```python
from build123d import *

# Parameters (mm, degrees)
EXTRUDE_1_DEPTH          = 660
CUT_EXTRUDE_1_DEPTH      = 661
CUT_EXTRUDE_1_DEPTH_BACK = 661
SHELL_1_T                = 10


with BuildPart() as part:
    # 草图1 → 凸台-拉伸1 (new body, symmetric)
    with BuildSketch(Plane(origin=(0, 0, 0), x_dir=(1, 0, 0), z_dir=(0, 1, 0))):
        Polygon((395, 8.660254038), (205, 337.749907476), (190, 346.410161514), (-190, 346.410161514), (-205, 337.749907476), (-395, 8.660254038), (-395, -8.660254038), (-205, -337.749907476), (-190, -346.410161514), (190, -346.410161514), (205, -337.749907476), (395, -8.660254038), align=None)
    extrude(amount=EXTRUDE_1_DEPTH, both=True)

    # 草图4 → 切除-拉伸1 (cut, two sides)
    with BuildSketch(Plane(origin=(0, 0, 0), x_dir=(1, 0, 0), z_dir=(0, 1, 0))) as cut_extrude_1_sk:
        with BuildLine():
            Line((190, 369.620348729), (190, 346.410161514))
            Line((190, 346.410161514), (11.76, 310.784114995))
            ThreePointArc((11.76, 310.784114995), (0, 309.620348729), (-11.76, 310.784114995))
            Line((-11.76, 310.784114995), (-190, 346.410161514))
            Line((-190, 346.410161514), (-190, 369.620348729))
            Line((-190, 369.620348729), (-190, 392.830535944))
            Line((-190, 392.830535944), (-11.76, 428.456582463))
            ThreePointArc((-11.76, 428.456582463), (0, 429.620348729), (11.76, 428.456582463))
            Line((11.76, 428.456582463), (190, 392.830535944))
            Line((190, 392.830535944), (190, 369.620348729))
        make_face()
        with BuildLine():
            Line((415.100611755, 20.265347645), (395, 8.660254038))
            Line((395, 8.660254038), (275.026938678, 145.207598749))
            ThreePointArc((275.026938678, 145.207598749), (268.139087528, 154.810174364), (263.266938678, 165.576516246))
            Line((263.266938678, 165.576516246), (205, 337.749907476))
            Line((205, 337.749907476), (225.100611755, 349.355001084))
            Line((225.100611755, 349.355001084), (245.20122351, 360.960094691))
            Line((245.20122351, 360.960094691), (365.174284832, 224.41274998))
            ThreePointArc((365.174284832, 224.41274998), (372.062135982, 214.810174364), (376.934284832, 204.043832483))
            Line((376.934284832, 204.043832483), (435.20122351, 31.870441253))
            Line((435.20122351, 31.870441253), (415.100611755, 20.265347645))
        make_face()
        with BuildLine():
            Line((225.100611755, -349.355001084), (205, -337.749907476))
            Line((205, -337.749907476), (263.266938678, -165.576516246))
            ThreePointArc((263.266938678, -165.576516246), (268.139087528, -154.810174364), (275.026938678, -145.207598749))
            Line((275.026938678, -145.207598749), (395, -8.660254038))
            Line((395, -8.660254038), (415.100611755, -20.265347645))
            Line((415.100611755, -20.265347645), (435.20122351, -31.870441253))
            Line((435.20122351, -31.870441253), (376.934284832, -204.043832483))
            ThreePointArc((376.934284832, -204.043832483), (372.062135982, -214.810174364), (365.174284832, -224.41274998))
            Line((365.174284832, -224.41274998), (245.20122351, -360.960094691))
            Line((245.20122351, -360.960094691), (225.100611755, -349.355001084))
        make_face()
        with BuildLine():
            Line((-190, -369.620348729), (-190, -346.410161514))
            Line((-190, -346.410161514), (-11.76, -310.784114995))
            ThreePointArc((-11.76, -310.784114995), (0, -309.620348729), (11.76, -310.784114995))
            Line((11.76, -310.784114995), (190, -346.410161514))
            Line((190, -346.410161514), (190, -369.620348729))
            Line((190, -369.620348729), (190, -392.830535944))
            Line((190, -392.830535944), (11.76, -428.456582463))
            ThreePointArc((11.76, -428.456582463), (0, -429.620348729), (-11.76, -428.456582463))
            Line((-11.76, -428.456582463), (-190, -392.830535944))
            Line((-190, -392.830535944), (-190, -369.620348729))
        make_face()
        with BuildLine():
            Line((-415.100611755, -20.265347645), (-395, -8.660254038))
            Line((-395, -8.660254038), (-275.026938678, -145.207598749))
            ThreePointArc((-275.026938678, -145.207598749), (-268.139087528, -154.810174364), (-263.266938678, -165.576516246))
            Line((-263.266938678, -165.576516246), (-205, -337.749907476))
            Line((-205, -337.749907476), (-225.100611755, -349.355001084))
            Line((-225.100611755, -349.355001084), (-245.20122351, -360.960094691))
            Line((-245.20122351, -360.960094691), (-365.174284832, -224.41274998))
            ThreePointArc((-365.174284832, -224.41274998), (-372.062135982, -214.810174364), (-376.934284832, -204.043832483))
            Line((-376.934284832, -204.043832483), (-435.20122351, -31.870441253))
            Line((-435.20122351, -31.870441253), (-415.100611755, -20.265347645))
        make_face()
        with BuildLine():
            Line((-225.100611755, 349.355001084), (-205, 337.749907476))
            Line((-205, 337.749907476), (-263.266938678, 165.576516246))
            ThreePointArc((-263.266938678, 165.576516246), (-268.139087528, 154.810174364), (-275.026938678, 145.207598749))
            Line((-275.026938678, 145.207598749), (-395, 8.660254038))
            Line((-395, 8.660254038), (-415.100611755, 20.265347645))
            Line((-415.100611755, 20.265347645), (-435.20122351, 31.870441253))
            Line((-435.20122351, 31.870441253), (-376.934284832, 204.043832483))
            ThreePointArc((-376.934284832, 204.043832483), (-372.062135982, 214.810174364), (-365.174284832, 224.41274998))
            Line((-365.174284832, 224.41274998), (-245.20122351, 360.960094691))
            Line((-245.20122351, 360.960094691), (-225.100611755, 349.355001084))
        make_face()
    extrude(amount=CUT_EXTRUDE_1_DEPTH, mode=Mode.SUBTRACT)
    extrude(cut_extrude_1_sk.sketch, amount=-CUT_EXTRUDE_1_DEPTH_BACK, mode=Mode.SUBTRACT)

    # 抽壳1 (no face opened: a closed hollow body)
    add(offset(amount=-SHELL_1_T, mode=Mode.PRIVATE), mode=Mode.SUBTRACT)


solid = part.part
```
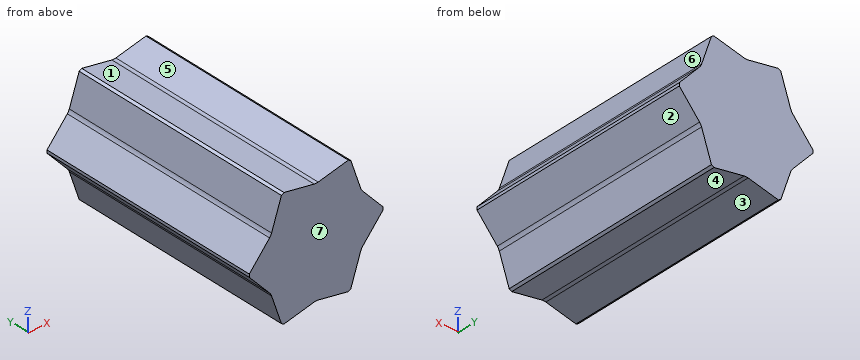
Check sheet for the modelled part. Datum: model origin and axes. Units: mm. Face numbers are marked on the shaded views. A direction names the side the tool comes from. Give positions to 0.01 mm unless a question says otherwise; leave off trailing zeros. Order: outer loops, then holes, each group sorted by start corner. A loop starts at its lowest first (then second) coordinate and runs counter-clockwise, first axis right, second up. Notation, with made-up numbers: (-22.75, -35.5) -> (-14.75, -35.5) arc R19 ccw to (-14.75, -9.5) -> close; hole circle Ø3 at (29, 0.25). An arc over 180 degrees is marked (long way). Use CSV: the item, a comma, the result in double quotes. Start each with the question number.
1) Material ranges on line 1 (Y direction, x = 195.5, z = -177.5); line 2 (X direction, y = 77, z = 289); line 3 (X direction, y = -560, z = 197), recorded low to high. Write a range as from..to.
2) Mould release check, pull along X, two halves, no side actions. Record for the marked faces 4, 5, 6 and 7: released by +X, released by -X, zero draft, split by the parting line, or undercut.
3) Set-up check for the marked faces 1, 2 and 3: record each of +Z, -Z, +X, -X, +Y, -Y from which the full face is reachable in a straight line by a thin tool's end or side.
4) Go/stop test with flat-tipped pins: P1, Ø3, axis at y = -180.5, z = 136, coming from the -X side; P2, Ø5, axis at y = 463.5, z = -219, coming from the +X side. Record where each tip stops, or that it passes through.
5) Sectioned sample at B-B, the plane x = 33.5. Record the boundary of the cut face in (y, z), plus the area to 3 significant figures.
6) Sectioned sample at A-A, the plane z = -101. Record the boundary of the cut face in (x, y).
Recorded:
1,line 1,"-660..-650, 650..660"
1,line 2,"-221.5..-210.94, 210.94..221.5"
1,line 3,"-252.63..-242.08, 242.08..252.63"
2,face 4,"undercut"
2,face 5,"undercut"
2,face 6,"released by +X"
2,face 7,"zero draft"
3,face 1,"+Z, +Y, -Y"
3,face 2,"-Z, +X, +Y, -Y"
3,face 3,"-Z, +Y, -Y"
4,P1,"x = -284.43"
4,P2,"x = 246.03"
5,outline,"(-660, -315.13) -> (660, -315.13) -> (660, 315.13) -> (-660, 315.13) -> close; hole (-650, -304.93) -> (650, -304.93) -> (650, 304.93) -> (-650, 304.93) -> close"
5,area,"39,100 mm2"
6,outline,"(-313.87, -660) -> (313.87, -660) -> (313.87, 660) -> (-313.87, 660) -> close; hole (-300.56, -650) -> (300.56, -650) -> (300.56, 650) -> (-300.56, 650) -> close"
